from build123d import *

# Parameters (mm, degrees)
FORO_3_0_3_2_D           = 3
FORO_3_0_3_2_DEPTH       = 8
FORO_3_0_3_2_TIP         = 0.901290929
SCHIZZO6_W               = 14.665621526
SCHIZZO6_H               = 2.346880268
TAGLIO_ESTRUSIONE1_DEPTH = 15


with BuildPart() as part:
    # Schizzo1 → Rivoluzione1 (revolve)
    with BuildSketch(Plane.XY):
        Polygon((15.282220449, 23.830923985), (-32.775254634, 23.830923985), (-32.775254634, 23.35027231), (-36.85329536, 23.35027231), (-36.85329536, 21.434825278), (-67.152934439, 21.434825278), (-67.152934439, 14.434825278), (-68.917878687, 14.434825278), (-68.917878687, 9.273654429), (-69.6840575, 9.273654429), (-69.6840575, 7.434825278), (-87.152934439, 7.434825278), (-87.152934439, 3.434825278), (15.282220449, 3.434825278), align=None)
    revolve(axis=Axis((15.282220449, 3.434825278, 0), (-1, 0, 0)))

    # Foro Ø3.0 (3)-2
    with Locations(Plane.ZY.offset(67.152934439)):
        with Locations((-9.915498688, 13.350323965), (9.915498688, 13.350323965), (9.915498688, -6.48067341), (-9.915498688, -6.48067341)):
            Hole(FORO_3_0_3_2_D / 2, depth=FORO_3_0_3_2_DEPTH)
            with Locations((0, 0, -(FORO_3_0_3_2_DEPTH + FORO_3_0_3_2_TIP / 2))):  # 118° drill point
                Cone(0, FORO_3_0_3_2_D / 2, FORO_3_0_3_2_TIP, mode=Mode.SUBTRACT)

    # Schizzo6 → Taglio-Estrusione1 (cut)
    with BuildSketch(Plane.ZY.offset(87.152934439)):
        with Locations((0.422032274, 6.608265412)):
            Rectangle(SCHIZZO6_W, SCHIZZO6_H)
    extrude(amount=-TAGLIO_ESTRUSIONE1_DEPTH, mode=Mode.SUBTRACT)


solid = part.part
Source: CAD feature listing. Evaluate the final solid. Frame: model axes, mm. A direction names the side the tool comes from. Coordinates: 2 decimals unless noted, no trailing zeros. Order: outer loops, then holes, each group sorted by start corner. A loop starts at its lowest first (then second) coordinate and runs counter-clockwise, first axis right, second up.
Item 1: Cut plane A-A (z = 0). Return loops of the section in (x, y).
Output values:
outline: (-87.15, -0.57) - (-69.68, -0.57) - (-69.68, -2.4) - (-68.92, -2.4) - (-68.92, -7.57) - (-67.15, -7.57) - (-67.15, -14.57) - (-36.85, -14.57) - (-36.85, -16.48) - (-32.78, -16.48) - (-32.78, -16.96) - (15.28, -16.96) - (15.28, 23.83) - (-32.78, 23.83) - (-32.78, 23.35) - (-36.85, 23.35) - (-36.85, 21.43) - (-67.15, 21.43) - (-67.15, 14.43) - (-68.92, 14.43) - (-68.92, 9.27) - (-69.68, 9.27) - (-69.68, 7.43) - (-72.15, 7.43) - (-72.15, 5.43) - (-87.15, 5.43) - close
Item 2: Cut plane B-B (y = -12.5). Return loops of the section in (x, z).
Output values:
outline: (-67.15, -8.37) - (-36.85, -8.37) - (-36.85, -11.95) - (-32.78, -11.95) - (-32.78, -12.73) - (15.28, -12.73) - (15.28, 12.73) - (-32.78, 12.73) - (-32.78, 11.95) - (-36.85, 11.95) - (-36.85, 8.37) - (-67.15, 8.37) - close
Item 3: Cut plane C-C (x = -7). Return loops of the section in (y, z).
Output values:
outline: circle Ø40.79 at (3.43, 0)
Item 4: Set-up query: faces 1 (the face through (15.282, 4, 0)), 2 (the face through (-69.684, 5, 4)), 3 (the face through (-72.153, 6, 0)). Return all of +Z, -Z, +X, -X, +Y, -Y with unobstructed straight access to the full face (end or side cutting, diameter ignored); none if empty.
Output values:
face 1: +Z, -Z, +X, +Y, -Y
face 2: -X
face 3: +Z, -Z, -X, +Y
Item 5: First-contact query: P1, Ø10, axis at x = -45.5, y = 6, coming from the -Z side; P2, Ø2, axis at y = 15.5, z = 9.5, coming from the -X side; P3, Ø3, axis at x = -5, z = -9, coming from the +Y side. Flat tips, straight axial feed; report the tip coordinate or a pass-through.
Output values:
P1: stops at z = -18
P2: stops at x = -67.15
P3: stops at y = 22.4
Item 6: Pull-direction query (Y, two-part tool) for faces 4 (the face through (-80, 5.435, 0)), 5 (the face through (-63.097, 13.801, -11.346)), 6 (the face through (-68.05, 1.05, 10.74)); classes: pulls with the +Y half, pulls with the -Y half, needs draft (parallel to the pull), parting line crosses it, or undercut.
Output values:
face 4: pulls with the +Y half
face 5: undercut
face 6: parting line crosses it
Item 7: Cut plane D-D (y = 19). Return loops of the section in (x, z).
Output values:
outline: (-67.15, -9.04) - (-36.85, -9.04) - (-36.85, -12.42) - (-32.78, -12.42) - (-32.78, -13.18) - (15.28, -13.18) - (15.28, 13.18) - (-32.78, 13.18) - (-32.78, 12.42) - (-36.85, 12.42) - (-36.85, 9.04) - (-67.15, 9.04) - close
Item 8: Material intervals for line 1 (X direction, y = 12, z = -16); line 2 (X direction, y = 15.5, z = -2.5); line 3 (Y direction, x = -18, z = 4), sorted ascending.
Output values:
line 1: x = -36.85 to 15.28
line 2: x = -67.15 to 15.28
line 3: y = -16.57 to 23.43
